Print and shaded views of the part. All mm, measured from the part's lowest x, y and z. A direction names the side the tool comes from. Coordinates: 2 decimals unless noted, no trailing zeros. Order: outer loops, then holes, each group sorted by start corner. A loop starts at its lowest first (then second) coordinate and runs counter-clockwise, first axis right, second up. Notation, with made-up numbers: (29.5, -7.75) -> (72.5, -7.75) arc R16 cw to (72.5, 0.25) -> close; hole circle Ø11 at (35.5, -36.75). An arc over 180 degrees is marked (long way). Write item = value, one per line. Start each with the question number.
Q1. Wall check: line 1 (X direction, y = 9, z = 8); line 2 (Y direction, x = 14.5, z = 9). Give the ranges that are in metal, low to high. Write a range as from..to.
Q2. Cut at C-C, the plane x = 13.75. List the corners of the cut face in (y, z), plus the area to 3 significant figures.
Q3. Flat gauge pins, fed straight in: pin 1 (4 mm diameter, centred on x = 3.5, y = 2.5, fed in from +Z); pin 2 (1.5 mm diameter, centred on x = 6.5, z = 9, fed in from +Y); pin 3 (1.5 mm diameter, centred on x = 12.5, y = 6.5, fed in from -Z); pin 4 (3 mm diameter, centred on x = 5.5, y = 13, fed in from +Z). Where does each tip first touch, or does it go through?
Q4. Mould opens along Y. For the marked faces 3, 4, 5 and 6 say: +Y half, -Y half, draft (parallel to the pull), parting line (faces both ways), or undercut.
Q5. Cut at B-B, the plane x = 8. List the corners of the cut face in (y, z).
Q6. Cut at A-A, the plane z = 8. List the corners of the cut face in (x, y).
Q7. Cut at D-D, the plane y = 14.75. List the corners of the cut face in (x, z), plus the area to 3 significant figures.
Q8. 3-axis set-ups, long thin cutter, end or side, ignore diameter. For the marked faces 1 and 2: which of +Z, -Z, +X, -X, +Y, -Y reach the whole face in a straight line?
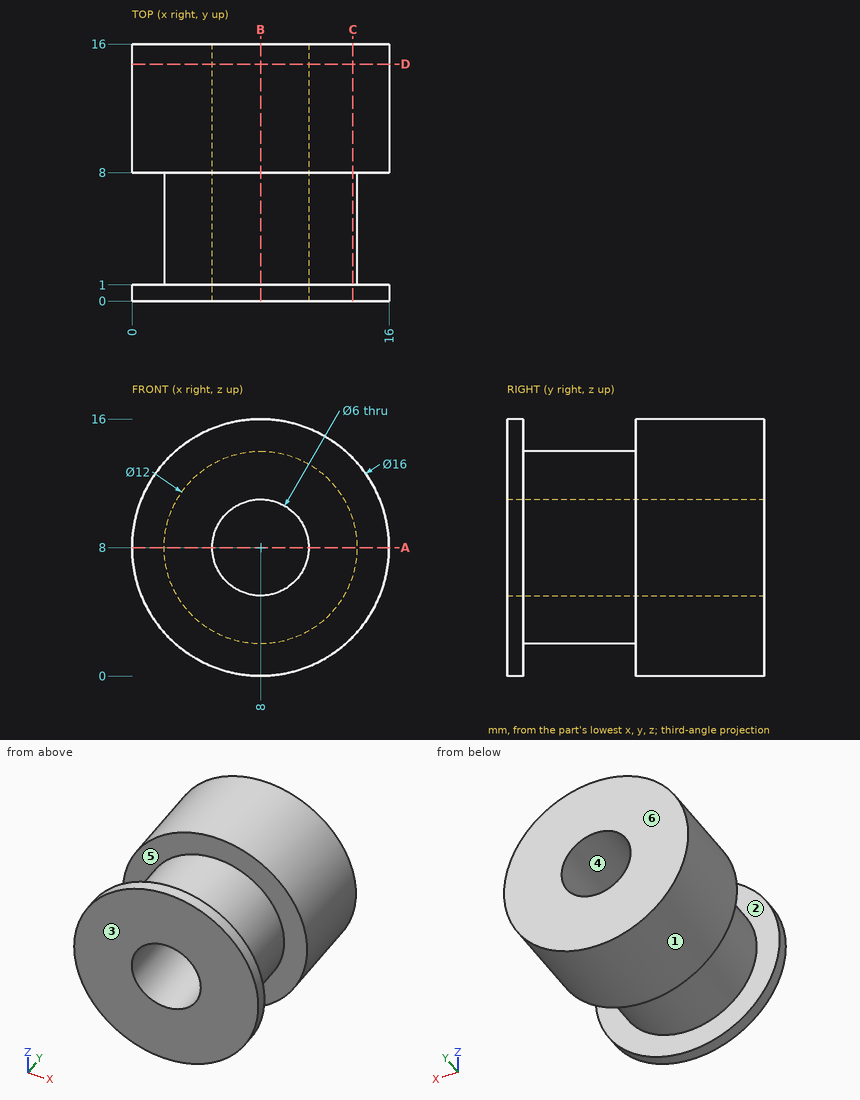
Here are the results:
q1.line_1 = 0..5, 11..16
q1.line_2 = 0..1, 8..16
q2.outline = (0, 2.44) -> (1, 2.44) -> (1, 6.29) -> (8, 6.29) -> (8, 2.44) -> (16, 2.44) -> (16, 13.56) -> (8, 13.56) -> (8, 9.71) -> (1, 9.71) -> (1, 13.56) -> (0, 13.56) -> close
q2.area = 124 mm²
q3.pin_1 = 15.34
q3.pin_2 = through
q3.pin_3 = 3.32
q3.pin_4 = 15.94
q4.face_3 = -Y half
q4.face_4 = draft
q4.face_5 = undercut
q4.face_6 = +Y half
q5.outline = (0, 0) -> (1, 0) -> (1, 2) -> (8, 2) -> (8, 0) -> (16, 0) -> (16, 5) -> (0, 5) -> close; (0, 11) -> (16, 11) -> (16, 16) -> (8, 16) -> (8, 14) -> (1, 14) -> (1, 16) -> (0, 16) -> close
q6.outline = (0, 0) -> (5, 0) -> (5, 16) -> (0, 16) -> (0, 8) -> (2, 8) -> (2, 1) -> (0, 1) -> close; (11, 0) -> (16, 0) -> (16, 1) -> (14, 1) -> (14, 8) -> (16, 8) -> (16, 16) -> (11, 16) -> close
q7.outline = circle Ø16 at (8, 8); hole circle Ø6 at (8, 8)
q7.area = 173 mm²
q8.face_1 = +Y, -Y
q8.face_2 = none
